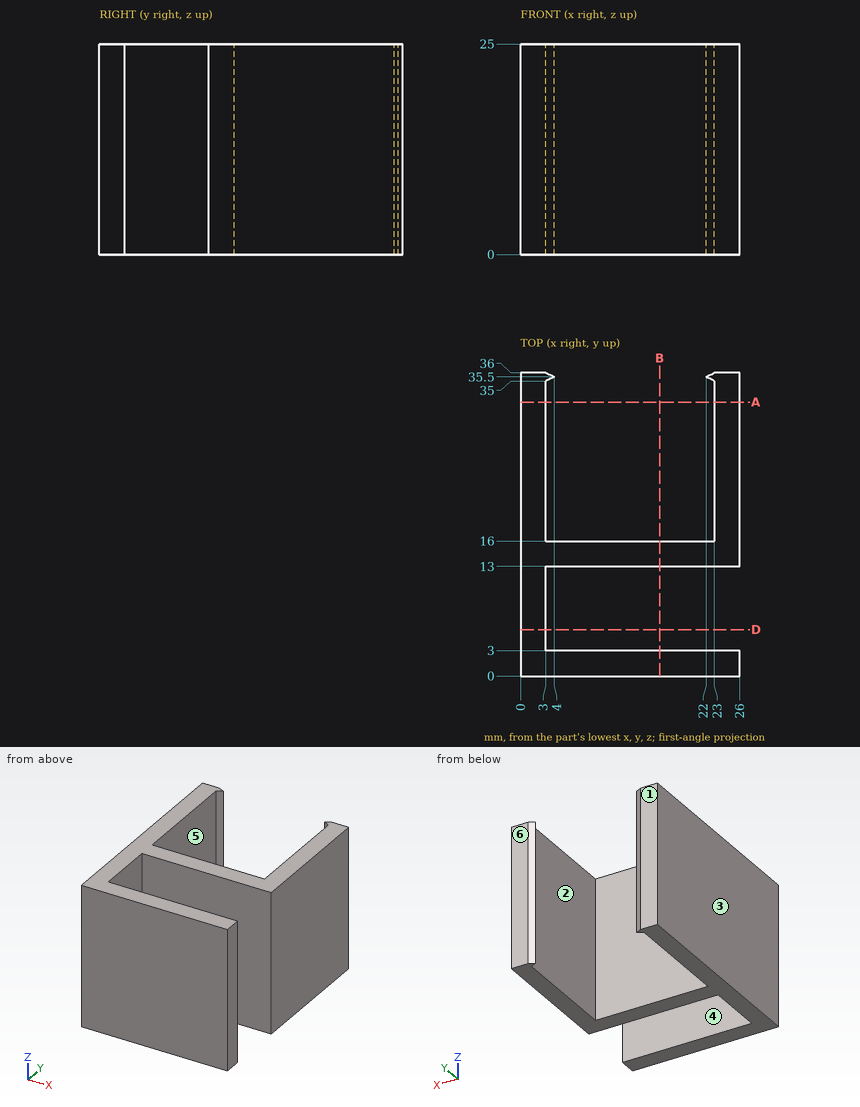
Verification items for this drawing (mm, ordinates from the low corner). A direction names the side the tool comes from. Give positions to 0.01 mm unless a question says otherwise; leave off trailing zeros. Loops run counter-clockwise (first coordinate to the right, second up) from the corner with the lowest first, then second, coordinate; pieces in that order, holes last. Notation, with made-up numbers: (-37, 36) - (10, 36) arc R16 cw to (10, 40) - close; hole circle Ø8 at (74, 16.5). An arc over 180 degrees is marked (long way). Write item = value, one per line. Start each with the question number.
Q1. Cross-section at B-B, the plane x = 16.5. Enter the section's corners in (y, z).
Q2. Tool access check on the marked faces 4, 5 and 6. Record the directions out of +Z, -Z, +X, -X, +Y, -Y that give a thin tool (end or side, any length) a straight path to the whole face; none if there is none.
Q3. Mould release check, pull along X, two halves, no side actions. Record for the marked faces 1, 2 and 3: released by +X, released by -X, zero draft, split by the parting line, or undercut.
Q4. Cross-section at D-D, the plane y = 5.5. Enter the section's corners in (x, z), and give its area (3 significant figures).
Q5. Depth check by flat-ended pin: P1, Ø6, axis at x = 13, z = 19.5, coming from the +Y side; P2, Ø3, axis at y = 9, z = 16, coming from the +X side. Enter the tip coordinate at first touch or a pass-through.
Q6. Thickness scan on line 1 (X direction, y = 26, z = 11); line 2 (Y direction, x = 18.5, z = 8); line 3 (Y direction, x = 3.5, z = 18.75). Record the ranges inside material, lowest first.
Q7. Cross-section at A-A, the plane y = 32.5. Enter the section's corners in (x, z).
Answer key:
q1.outline = (0, 0) - (3, 0) - (3, 25) - (0, 25) - close; (13, 0) - (16, 0) - (16, 25) - (13, 25) - close
q2.face_4 = +Z, -Z, +X
q2.face_5 = +Z, -Z
q2.face_6 = +Z, -Z, +X, -X, +Y
q3.face_1 = zero draft
q3.face_2 = undercut
q3.face_3 = released by -X
q4.outline = (0, 0) - (3, 0) - (3, 25) - (0, 25) - close
q4.area = 75.0 mm^2
q5.P1 = 16
q5.P2 = 3
q6.line_1 = 0 to 3, 23 to 26
q6.line_2 = 0 to 3, 13 to 16
q6.line_3 = 0 to 3, 13 to 16, 35.25 to 35.75
q7.outline = (0, 0) - (3, 0) - (3, 25) - (0, 25) - close; (23, 0) - (26, 0) - (26, 25) - (23, 25) - close
